Read the model definition and answer for the solid it produces. Units are mm, in the model's axes. A direction names the side the tool comes from. Coordinates: 2 decimals unless noted, no trailing zeros. Loops run counter-clockwise (first coordinate to the right, second up) from the corner with the lowest first, then second, coordinate; pieces in that order, holes last. Notation, with made-up numbers: M 36,3.25 L 78,3.25 A20 cw 78,9.25 Z; hole C 23.25,-0.75 d10. An arc over 180 degrees is marked long. Put each result on its own line as item: value.
from build123d import *

# Parameters (mm, degrees)
SKETCH2_R           = 25.4
SKETCH2_R_2         = 4.7625
SKETCH2_R_3         = 7.14375
BOSS_EXTRUDE1_DEPTH = 17.4625
SKETCH2_4_R         = 25.4
SKETCH2_4_R_2       = 14.2875
SKETCH2_4_R_3       = 4.7625
BOSS_EXTRUDE2_DEPTH = 19.05
SKETCH2_5_R         = 38.1
SKETCH2_5_R_2       = 25.4
BOSS_EXTRUDE3_DEPTH = 63.5
SKETCH4_R           = 34.925
SKETCH4_R_2         = 22.225
BOSS_EXTRUDE4_DEPTH = 19.05
SKETCH4_5_R         = 34.925
SKETCH4_5_R_2       = 22.225
BOSS_EXTRUDE5_DEPTH = 41.275
RIB1_REACH          = 322.848
SKETCH5_WALL_W      = 733.847979228
SKETCH5_WALL_H      = 12.7
RIB2_REACH          = 282.408
SKETCH6_WALL_W      = 630.127475074
SKETCH6_WALL_H      = 12.7
RIB3_REACH          = 282.408
SKETCH7_WALL_W      = 618.773406406
SKETCH7_WALL_H      = 12.7


with BuildPart() as part:
    # Sketch2 → Boss-Extrude1 (new body)
    with BuildSketch(Plane(origin=(0, 0, 0), x_dir=(1, 0, 0), z_dir=(0, 1, 0))):
        with BuildLine():
            ThreePointArc((38.1, 0), (0.952797982, 38.088084436), (-38.052345197, 1.905))
            ThreePointArc((-38.052345197, 1.905), (-65.571053954, -58.064169637), (-126.841150657, -82.55))
            Line((-126.841150657, -82.55), (-222.25, -82.55))
            ThreePointArc((-222.25, -82.55), (-241.02652856, -98.383717171), (-228.590223243, -119.563965855))
            Line((-228.590223243, -119.563965855), (-120.640223243, -157.663965855))
            ThreePointArc((-120.640223243, -157.663965855), (-117.516282829, -158.47652856), (-114.3, -158.75))
            Line((-114.3, -158.75), (19.05, -158.75))
            ThreePointArc((19.05, -158.75), (32.520384182, -153.170384182), (38.1, -139.7))
            Line((38.1, -139.7), (38.1, 0))
        make_face()
        with Locations(Location((0, 0, 0), (0, 0, 270))):
            Circle(SKETCH2_R, mode=Mode.SUBTRACT)
        with Locations(Location((-19.05, -139.7, 0), (0, 0, 270))):
            Circle(SKETCH2_R_2, mode=Mode.SUBTRACT)
        with Locations(Location((-222.25, -101.6, 0), (0, 0, 270))):
            Circle(SKETCH2_R_3, mode=Mode.SUBTRACT)
        with Locations(Location((-114.3, -139.7, 0), (0, 0, 270))):
            Circle(SKETCH2_R_3, mode=Mode.SUBTRACT)
        with Locations(Location((19.05, -139.7, 0), (0, 0, 270))):
            Circle(SKETCH2_R_3, mode=Mode.SUBTRACT)
        with Locations(Location((-44.45, -98.425, 0), (0, 0, 270))):
            Circle(SKETCH2_R_3, mode=Mode.SUBTRACT)
    extrude(amount=BOSS_EXTRUDE1_DEPTH)

    # Sketch2_4 → Boss-Extrude2 (add)
    with BuildSketch(Plane(origin=(0, 0, 0), x_dir=(1, 0, 0), z_dir=(0, 1, 0))):
        with BuildLine():
            ThreePointArc((38.1, 0), (0.952797982, 38.088084436), (-38.052345197, 1.905))
            ThreePointArc((-38.052345197, 1.905), (-65.571053954, -58.064169637), (-126.841150657, -82.55))
            Line((-126.841150657, -82.55), (-222.25, -82.55))
            ThreePointArc((-222.25, -82.55), (-241.02652856, -98.383717171), (-228.590223243, -119.563965855))
            Line((-228.590223243, -119.563965855), (-120.640223243, -157.663965855))
            ThreePointArc((-120.640223243, -157.663965855), (-117.516282829, -158.47652856), (-114.3, -158.75))
            Line((-114.3, -158.75), (19.05, -158.75))
            ThreePointArc((19.05, -158.75), (32.520384182, -153.170384182), (38.1, -139.7))
            Line((38.1, -139.7), (38.1, 0))
        make_face()
        with Locations(Location((0, 0, 0), (0, 0, 270))):
            Circle(SKETCH2_4_R, mode=Mode.SUBTRACT)
        with Locations(Location((-44.45, -98.425, 0), (0, 0, 90))):
            Circle(SKETCH2_4_R_2, mode=Mode.SUBTRACT)
        with Locations(Location((-114.3, -139.7, 0), (0, 0, 90))):
            Circle(SKETCH2_4_R_2, mode=Mode.SUBTRACT)
        with Locations(Location((-222.25, -101.6, 0), (0, 0, 90))):
            Circle(SKETCH2_4_R_2, mode=Mode.SUBTRACT)
        with Locations(Location((-19.05, -139.7, 0), (0, 0, 270))):
            Circle(SKETCH2_4_R_3, mode=Mode.SUBTRACT)
        with Locations(Location((19.05, -139.7, 0), (0, 0, 90))):
            Circle(SKETCH2_4_R_2, mode=Mode.SUBTRACT)
    extrude(amount=BOSS_EXTRUDE2_DEPTH)

    # Sketch2_5 → Boss-Extrude3 (add)
    with BuildSketch(Plane(origin=(0, 0, 0), x_dir=(1, 0, 0), z_dir=(0, 1, 0))):
        with Locations(Location((0, 0, 0), (0, 0, 177.134016017))):
            Circle(SKETCH2_5_R)
        with Locations(Location((0, 0, 0), (0, 0, 270))):
            Circle(SKETCH2_5_R_2, mode=Mode.SUBTRACT)
    extrude(amount=BOSS_EXTRUDE3_DEPTH)

    # Sketch4 → Boss-Extrude4 (add)
    with BuildSketch(Plane(origin=(0, 0, 82.55), x_dir=(-1, 0, 0), z_dir=(0, 0, -1))):
        with BuildLine():
            Line((201.684846649, 19.05), (180.079874513, 112.631415573))
            ThreePointArc((180.079874513, 112.631415573), (180.75049706, 108.728622241), (180.975, 104.775))
            ThreePointArc((180.975, 104.775), (142.096377759, 70.07450294), (112.020125487, 112.631415573))
            Line((112.020125487, 112.631415573), (90.415153351, 19.05))
            Line((90.415153351, 19.05), (126.841150657, 19.05))
            Line((126.841150657, 19.05), (201.684846649, 19.05))
        make_face()
        with Locations((146.05, 104.775)):
            Circle(SKETCH4_R)
        with Locations((146.05, 104.775)):
            Circle(SKETCH4_R_2, mode=Mode.SUBTRACT)
    extrude(amount=-BOSS_EXTRUDE4_DEPTH)

    # Sketch4_5 → Boss-Extrude5 (add)
    with BuildSketch(Plane(origin=(0, 0, 82.55), x_dir=(-1, 0, 0), z_dir=(0, 0, -1))):
        with Locations((146.05, 104.775)):
            Circle(SKETCH4_5_R)
        with Locations((146.05, 104.775)):
            Circle(SKETCH4_5_R_2, mode=Mode.SUBTRACT)
    extrude(amount=BOSS_EXTRUDE5_DEPTH)

    # Sketch5 wall → Rib1 (add, up to next)
    with BuildSketch(Plane(origin=(0, 38.1, 78.952856836), x_dir=(0, -0.422618261742, 0.906307787036), z_dir=(0, -0.906307787036, -0.422618261742)), mode=Mode.PRIVATE) as rib1_sk1:
        Rectangle(SKETCH5_WALL_W, SKETCH5_WALL_H)
    rib1_tool1 = extrude(rib1_sk1.sketch, amount=RIB1_REACH, mode=Mode.PRIVATE) - part.part
    add(rib1_tool1.solids().sort_by_distance((0, 38.1, 78.952856836))[0])

    # Sketch6 wall → Rib2 (add, up to next)
    with BuildSketch(Plane(origin=(-146.05, 44.45, 123.67988314), x_dir=(0, 0.754709580223, -0.65605902899), z_dir=(0, 0.65605902899, 0.754709580223)), mode=Mode.PRIVATE) as rib2_sk1:
        Rectangle(SKETCH6_WALL_W, SKETCH6_WALL_H)
    rib2_tool1 = extrude(rib2_sk1.sketch, amount=-RIB2_REACH, mode=Mode.PRIVATE) - part.part
    add(rib2_tool1.solids().sort_by_distance((-146.05, 44.45, 123.67988314))[0])

    # Sketch7 wall → Rib3 (add, up to next)
    with BuildSketch(Plane(origin=(-146.05, 44.45, 70.818630511), x_dir=(0, 0.907846577763, -0.41930250565), z_dir=(0, 0.41930250565, 0.907846577763)), mode=Mode.PRIVATE) as rib3_sk1:
        Rectangle(SKETCH7_WALL_W, SKETCH7_WALL_H)
    rib3_tool1 = extrude(rib3_sk1.sketch, amount=RIB3_REACH, mode=Mode.PRIVATE) - part.part
    add(rib3_tool1.solids().sort_by_distance((-146.05, 44.45, 70.818630511))[0])


solid = part.part
1) Find section A-A, the plane y = 49. Write down the section's boundary in (x, z).
Answer list:
outline: M -194.77,82.55 L -152.4,82.55 L -152.4,68.72 L -139.7,68.72 L -139.7,82.55 L -97.33,82.55 L -97.33,101.6 L -139.7,101.6 L -139.7,119.72 L -152.4,119.72 L -152.4,101.6 L -194.77,101.6 Z; M -6.35,37.57 A38.1 ccw long 6.35,37.57 L 6.35,55.58 L -6.35,55.58 Z; hole C 0,0 d50.8
2) Straight lines are drawn through the part: line 1 (X direction, y = 18, z = 101); line 2 (X direction, y = 8.5, z = 101.6); line 3 (Y direction, x = -42, z = 115.5). For each, find the intervals that lie inside material, in ascending order. Write a range as [from, to].
Answer list:
line 1: x = [-241.29, -236.52], [-207.98, -58.5], [-30.4, 38.1]
line 2: x = [-241.3, -229.39], [-215.11, -50.85], [-38.05, 38.1]
line 3: y = [0, 19.05]
3) Which of the six approach directions +Z, -Z, +X, -X, +Y, -Y give full straight-line access (tool end or side, diameter ignored) to faces 4 (the flat face through (12, 17.462, 143)), 5 (the flat face through (-146.14, 44.38, 70.85)), 6 (the flat face through (-0.089, 38.493, 78.111))?
Answer list:
face 4: +Y
face 5: -Z, -X, -Y
face 6: +Z, +X, +Y
4) Find section B-B, the plane x = 0. Write down the section's boundary in (y, z), plus the area to 3 significant figures.
Answer list:
outline: M 0,-38.1 L 63.5,-38.1 L 63.5,-25.4 L 0,-25.4 Z; M 0,25.4 L 63.5,25.4 L 63.5,38.1 L 57.15,38.1 L 19.05,119.81 L 19.05,158.75 L 0,158.75 Z
area: 5,470 mm^2
5) Determine the mould class of faces 1 (the flat face through (-73, 0, 81)), 2 (the cylindrical face through (-18.841, 9.392, 134.942)), 3 (the flat face through (-152.4, 54, 76)) for opening direction X: released by +X, released by -X, zero draft, split by the parting line, or undercut.
Answer list:
face 1: zero draft
face 2: undercut
face 3: released by -X
6) Find section C-C, the plane z = 5. Write down the section's boundary in (x, y), plus the area to 3 significant figures.
Answer list:
outline: M -38.67,0 L -24.9,0 L -24.9,63.5 L -37.77,63.5 L -37.77,19.05 L -38.67,19.05 Z; M 24.9,0 L 38.1,0 L 38.1,19.05 L 37.77,19.05 L 37.77,63.5 L 24.9,63.5 Z
area: 1,660 mm^2
7) Find section D-D, the plane y = 12.5. Count the separate pieces of the cut face and the enclosed holes in it, plus the area to 3 significant figures.
Answer list:
separate pieces: 1
enclosed holes: 6
area: 25,900 mm^2
8) Given pin 1 Ø6 at (y, z) = (36, 65) entering from +X; pin 2 Ø18.5 at (x, z) = (-44.45, 98.425) entering from +Y; pin 3 Ø5 at (y, z) = (31.5, 25) entering from +X, each flat-ended and moving along its own axis, determine where each tip first touches the part or whether it passes through.
Answer list:
pin 1: stops at x = 6.35
pin 2: stops at y = 17.46
pin 3: stops at x = 30.75
